```python
from build123d import *

# Parameters (mm, degrees)
SKETCH1_W                                  = 18
SKETCH1_H                                  = 20
BOSS_EXTRUDE1_DEPTH                        = 2.5
SKETCH2_W                                  = 18
SKETCH2_H                                  = 5
BOSS_EXTRUDE2_DEPTH                        = 42
SKETCH7_W                                  = 18
SKETCH7_H                                  = 5
BOSS_EXTRUDE3_DEPTH                        = 42
CSK_FOR_M3_HEX_SOCKET_COUNTERSUNK_CAP_SC_D = 4.2
SKETCH10_W                                 = 18
SKETCH10_H                                 = 42
BOSS_EXTRUDE4_DEPTH                        = 6
SKETCH9_W                                  = 6.5
SKETCH9_H                                  = 6.5
CUT_EXTRUDE2_DEPTH                         = 52.01225343
TAPPED_HOLE_FOR_M4X0_7_HELICOIL1_D         = 4.2
TAPPED_HOLE_FOR_M4X0_7_HELICOIL1_DEPTH     = 11
SKETCH11_R                                 = 2
CUT_EXTRUDE3_DEPTH                         = 6
FILLET1_R                                  = 2.5


with BuildPart() as part:
    # Sketch1 → Boss-Extrude1 (new, symmetric)
    with BuildSketch(Plane.XY):
        Rectangle(SKETCH1_W, SKETCH1_H)
    extrude(amount=BOSS_EXTRUDE1_DEPTH, both=True)

    # Sketch2 → Boss-Extrude2 (add)
    with BuildSketch(Plane(origin=(0, 0, 2.5), x_dir=(-1, 0, 0), z_dir=(0, 0, -1))):
        with Locations((0, -7.5)):
            Rectangle(SKETCH2_W, SKETCH2_H)
    extrude(amount=BOSS_EXTRUDE2_DEPTH)

    # Sketch7 → Boss-Extrude3 (add)
    with BuildSketch(Plane.XY.offset(2.5)):
        with Locations((0, 12.5)):
            Rectangle(SKETCH7_W, SKETCH7_H)
    extrude(amount=-BOSS_EXTRUDE3_DEPTH)

    # CSK for M3 Hex Socket Countersunk Cap Screw1 (through all)
    with Locations(Plane.XY.offset(2.5)):
        with Locations((-5, 2.5), (5, 2.5)):
            Hole(CSK_FOR_M3_HEX_SOCKET_COUNTERSUNK_CAP_SC_D / 2)

    # Sketch10 → Boss-Extrude4 (add)
    with BuildSketch(Plane.XZ.offset(10)):
        with Locations((0, -18.5)):
            Rectangle(SKETCH10_W, SKETCH10_H)
    extrude(amount=BOSS_EXTRUDE4_DEPTH)

    # Sketch9 → Cut-Extrude2 (cut, through all)
    with BuildSketch(Plane.XZ.offset(16)):
        with Locations((-5.75, -36.25)):
            Rectangle(SKETCH9_W, SKETCH9_H)
    extrude(amount=-CUT_EXTRUDE2_DEPTH, mode=Mode.SUBTRACT)

    # Tapped Hole for M4x0.7 Helicoil1
    with Locations(Plane(origin=(0, -16, 0), x_dir=(-1, 0, 0), z_dir=(0, -1, 0))):
        with Locations((-4, 28.375), (-4, 8.375)):
            Hole(TAPPED_HOLE_FOR_M4X0_7_HELICOIL1_D / 2, depth=TAPPED_HOLE_FOR_M4X0_7_HELICOIL1_DEPTH)

    # Sketch11 → Cut-Extrude3 (cut)
    with BuildSketch(Plane(origin=(0, -16, 0), x_dir=(-1, 0, 0), z_dir=(0, -1, 0))):
        with Locations(Location((4, 8.375, 0), (0, 0, 90))):
            Circle(SKETCH11_R)
    extrude(amount=-CUT_EXTRUDE3_DEPTH, mode=Mode.SUBTRACT)

    # Fillet1
    fillet1_edges = [part.edges().sort_by_distance(p)[0] for p in [
        (0, -5, -2.5),
        (0, 10, -2.5),
    ]]
    fillet(fillet1_edges, radius=FILLET1_R)


solid = part.part
```
Build history of the part. All positions in model axes, mm. A direction names the side the tool comes from. Give positions to 0.01 mm unless a question says otherwise; leave off trailing zeros. Loops run counter-clockwise (first coordinate to the right, second up) from the corner with the lowest first, then second, coordinate; pieces in that order, holes last. Notation, with made-up numbers: (29.5, 88) - (39.5, 88) arc R6 ccw to (39.5, 92) - close; hole circle Ø11 at (27, 88). An arc over 180 degrees is marked (long way). Use a Markdown table: item, result.
(1) Wall check: line 1 along Z through (x, y) = (4, -10.5) (3 decimals); line 2 along Y through (x, z) = (-3.5, -10); line 3 along Y through (x, z) = (-1, -8.5). Give the ranges that are in metal, low to high.
Taken from the geometry:
| item | result |
|---|---|
| line 1 | -39.5 to -30.475, -26.275 to -10.475, -6.275 to 2.5 |
| line 2 | -10 to -5, 10 to 15 |
| line 3 | -16 to -5, 10 to 15 |
(2) Band-saw the part on C-C (x = 4). Give the cut face in (y, z) (3 decimals), and give its area (3 significant figures).
Taken from the geometry:
| item | result |
|---|---|
| outline | (-16, -39.5) - (-5, -39.5) - (-5, -30.475) - (-16, -30.475) - close; (-16, -26.275) - (-5, -26.275) - (-5, -10.475) - (-16, -10.475) - close; (-16, -6.275) - (-5, -6.275) - (-5, -5) arc R2.5 cw to (-2.5, -2.5) - (0.653, -2.5) - (0.653, 2.5) - (-16, 2.5) - close; (4.347, -2.5) - (7.5, -2.5) arc R2.5 cw to (10, -5) - (10, -39.5) - (15, -39.5) - (15, 2.5) - (4.347, 2.5) - close |
| area | 639 mm2 |
(3) Drop flat-ended pins along their axis: pin 1 Ø4 at (x, y) = (-5, 2.5) entering from -Z; pin 2 Ø1.5 at (y, z) = (11.5, -37.5) entering from -X; pin 3 Ø8 at (x, y) = (-0.5, 0.5) entering from -Z; pin 4 Ø5 at (x, y) = (5, 2.5) entering from -Z. Give the stop position or say it passes through.
Taken from the geometry:
| item | result |
|---|---|
| pin 1 | through |
| pin 2 | x = -2.5 |
| pin 3 | z = -2.71 |
| pin 4 | z = -2.5 |
(4) Band-saw the part on B-B (z = -24.5). Give the cut face in (x, y).
Taken from the geometry:
| item | result |
|---|---|
| outline | (-9, -16) - (9, -16) - (9, -5) - (-9, -5) - close; (-9, 10) - (9, 10) - (9, 15) - (-9, 15) - close |
(5) Band-saw the part on D-D (x = -4). Give the cut face in (y, z) (3 decimals).
Taken from the geometry:
| item | result |
|---|---|
| outline | (-16, -33) - (-5, -33) - (-5, -5) arc R2.5 cw to (-2.5, -2.5) - (0.653, -2.5) - (0.653, 2.5) - (-16, 2.5) - (-16, -6.375) - (-10, -6.375) - (-10, -10.375) - (-16, -10.375) - close; (4.347, -2.5) - (7.5, -2.5) arc R2.5 cw to (10, -5) - (10, -33) - (15, -33) - (15, 2.5) - (4.347, 2.5) - close |
(6) Pull direction X, two halves, no side cores. Call faces 1 (the face through (0, 0, 2.5)), 2 (the face through (-4, -10, -8)), 3 (the face through (-2.5, -11, -36)), 4 (the face through (6, -10.42, -29.01)): +X half, -X half, draft (parallel to the pull), parting line (faces both ways), or undercut.
Taken from the geometry:
| item | result |
|---|---|
| face 1 | draft |
| face 2 | undercut |
| face 3 | -X half |
| face 4 | undercut |
(7) Band-saw the part on A-A (y = 2.5). Give the cut face in (x, z), and give its area (3 significant figures).
Taken from the geometry:
| item | result |
|---|---|
| outline | (-9, -2.5) - (-7.1, -2.5) - (-7.1, 2.5) - (-9, 2.5) - close; (-2.9, -2.5) - (2.9, -2.5) - (2.9, 2.5) - (-2.9, 2.5) - close; (7.1, -2.5) - (9, -2.5) - (9, 2.5) - (7.1, 2.5) - close |
| area | 48.0 mm2 |
(8) Which spindle directions (+Z, -Z, +X, -X, +Y, -Y) get a long thin tool onto all of the face, cutting with end or side? Do faces 5 (the face through (3, 13, -39.5)), 6 (the face through (0, 9, -3)), 7 (the face through (-6, -11, -33)), 8 (the face through (3.727, -10.423, -10.457)). Say none if no direction does.
Taken from the geometry:
| item | result |
|---|---|
| face 5 | -Z, +X, -X, +Y, -Y |
| face 6 | -Z, +X, -X |
| face 7 | -Z, -X, +Y, -Y |
| face 8 | -Y |
